Here's how the part is built. I have some questions about the finished solid (model axes, mm). Round coordinates to 2 decimals unless told otherwise and drop trailing zeros. Order: outer loops, then holes, each group sorted by start corner. A loop starts at its lowest first (then second) coordinate and runs counter-clockwise, first axis right, second up. Notation, with made-up numbers: M 85,-19 L 89,-19 A24 ccw 89,10 Z; hole C 84,53.25 d11. An arc over 180 degrees is marked long. Answer as CSV lines item,"result". Start each with the question number.
```python
from build123d import *

# Parameters (mm, degrees)
SKETCH1_W               = 283
SKETCH1_H               = 135
SKETCH1_R               = 1.75
BOSS_EXTRUDE1_DEPTH     = 4.5
SKETCH1_3_R             = 1.75
CUT_EXTRUDE1_DEPTH      = 4.5
MIRROR3_COPY_1_SKETCH_R = 1.75
MIRROR3_COPY_1_DEPTH    = 4.5
CUT_EXTRUDE2_REACH      = 6.5
SKETCH2_R               = 1.75
CUT_EXTRUDE3_REACH      = 6.5
SKETCH3_R               = 32.95
SKETCH3_R_2             = 14.5
SKETCH3_R_3             = 2.5


with BuildPart() as part:
    # Sketch1 → Boss-Extrude1 (new body)
    with BuildSketch(Plane.XY):
        Rectangle(SKETCH1_W, SKETCH1_H)
        with Locations((-131.5, 57.5)):
            Circle(SKETCH1_R, mode=Mode.SUBTRACT)
        with Locations((-131.5, 57.5)):
            Circle(SKETCH1_R)
    extrude(amount=BOSS_EXTRUDE1_DEPTH)

    # Sketch1_3 → Cut-Extrude1 (cut)
    with BuildSketch(Plane.XY):
        with Locations((-131.5, 57.5)):
            Circle(SKETCH1_3_R)
    cut_extrude1 = extrude(amount=CUT_EXTRUDE1_DEPTH, mode=Mode.SUBTRACT)

    # Mirror2: Cut-Extrude1 across plane
    add(cut_extrude1.mirror(Plane.ZX), mode=Mode.SUBTRACT)

    # Mirror3: Cut-Extrude1 across plane
    add(cut_extrude1.mirror(Plane(origin=(0, 0, 0), x_dir=(0, 0, 1), z_dir=(1, 0, 0))), mode=Mode.SUBTRACT)

    # Mirror3 copy 1 sketch → Mirror3 copy 1 (cut)
    with BuildSketch(Plane(origin=(0, 0, 0), x_dir=(-1, 0, 0), z_dir=(0, 0, 1))):
        with Locations((-131.5, 57.5)):
            Circle(MIRROR3_COPY_1_SKETCH_R)
    extrude(amount=MIRROR3_COPY_1_DEPTH, mode=Mode.SUBTRACT)

    # Sketch2 → Cut-Extrude2 (cut, up to next)
    with BuildSketch(Plane.XY.offset(4.5), mode=Mode.PRIVATE) as cut_extrude2_sk1:
        with Locations((-87.5, -14)):
            Circle(SKETCH2_R)
    cut_extrude2_tool1 = extrude(cut_extrude2_sk1.sketch, amount=-CUT_EXTRUDE2_REACH, mode=Mode.PRIVATE) & part.part
    add(cut_extrude2_tool1.solids().sort_by_distance((-87.5, -14, 4.5))[0], mode=Mode.SUBTRACT)
    # Sketch2 → Cut-Extrude2 (cut, up to next)
    with BuildSketch(Plane.XY.offset(4.5), mode=Mode.PRIVATE) as cut_extrude2_sk2:
        with Locations((-115.5, -14)):
            Circle(SKETCH2_R)
    cut_extrude2_tool2 = extrude(cut_extrude2_sk2.sketch, amount=-CUT_EXTRUDE2_REACH, mode=Mode.PRIVATE) & part.part
    add(cut_extrude2_tool2.solids().sort_by_distance((-115.5, -14, 4.5))[0], mode=Mode.SUBTRACT)
    # Sketch2 → Cut-Extrude2 (cut, up to next)
    with BuildSketch(Plane.XY.offset(4.5), mode=Mode.PRIVATE) as cut_extrude2_sk3:
        with Locations((-115.5, 14)):
            Circle(SKETCH2_R)
    cut_extrude2_tool3 = extrude(cut_extrude2_sk3.sketch, amount=-CUT_EXTRUDE2_REACH, mode=Mode.PRIVATE) & part.part
    add(cut_extrude2_tool3.solids().sort_by_distance((-115.5, 14, 4.5))[0], mode=Mode.SUBTRACT)
    # Sketch2 → Cut-Extrude2 (cut, up to next)
    with BuildSketch(Plane.XY.offset(4.5), mode=Mode.PRIVATE) as cut_extrude2_sk4:
        with Locations((-87.5, 14)):
            Circle(SKETCH2_R)
    cut_extrude2_tool4 = extrude(cut_extrude2_sk4.sketch, amount=-CUT_EXTRUDE2_REACH, mode=Mode.PRIVATE) & part.part
    add(cut_extrude2_tool4.solids().sort_by_distance((-87.5, 14, 4.5))[0], mode=Mode.SUBTRACT)
    # Sketch2 → Cut-Extrude2 (cut, up to next)
    with BuildSketch(Plane.XY.offset(4.5), mode=Mode.PRIVATE) as cut_extrude2_sk5:
        with BuildLine():
            Line((-68.5, -5), (-68.5, 5))
            ThreePointArc((-68.5, 5), (-66.5, 7), (-64.5, 5))
            Line((-64.5, 5), (-64.5, -5))
            ThreePointArc((-64.5, -5), (-66.5, -7), (-68.5, -5))
        make_face()
    cut_extrude2_tool5 = extrude(cut_extrude2_sk5.sketch, amount=-CUT_EXTRUDE2_REACH, mode=Mode.PRIVATE) & part.part
    add(cut_extrude2_tool5.solids().sort_by_distance((-66.5, 0, 4.5))[0], mode=Mode.SUBTRACT)

    # Sketch3 → Cut-Extrude3 (cut, up to next)
    with BuildSketch(Plane.XY.offset(4.5), mode=Mode.PRIVATE) as cut_extrude3_sk1:
        with Locations((75, -2.5)):
            Circle(SKETCH3_R)
    cut_extrude3_tool1 = extrude(cut_extrude3_sk1.sketch, amount=-CUT_EXTRUDE3_REACH, mode=Mode.PRIVATE) & part.part
    add(cut_extrude3_tool1.solids().sort_by_distance((75, -2.5, 4.5))[0], mode=Mode.SUBTRACT)
    # Sketch3 → Cut-Extrude3 (cut, up to next)
    with BuildSketch(Plane.XY.offset(4.5), mode=Mode.PRIVATE) as cut_extrude3_sk2:
        Circle(SKETCH3_R_2)
    cut_extrude3_tool2 = extrude(cut_extrude3_sk2.sketch, amount=-CUT_EXTRUDE3_REACH, mode=Mode.PRIVATE) & part.part
    add(cut_extrude3_tool2.solids().sort_by_distance((0, 0, 4.5))[0], mode=Mode.SUBTRACT)
    # Sketch3 → Cut-Extrude3 (cut, up to next)
    with BuildSketch(Plane.XY.offset(4.5), mode=Mode.PRIVATE) as cut_extrude3_sk3:
        with Locations((-6.525, -30.95)):
            Circle(SKETCH3_R_3)
    cut_extrude3_tool3 = extrude(cut_extrude3_sk3.sketch, amount=-CUT_EXTRUDE3_REACH, mode=Mode.PRIVATE) & part.part
    add(cut_extrude3_tool3.solids().sort_by_distance((-6.525, -30.95, 4.5))[0], mode=Mode.SUBTRACT)
    # Sketch3 → Cut-Extrude3 (cut, up to next)
    with BuildSketch(Plane.XY.offset(4.5), mode=Mode.PRIVATE) as cut_extrude3_sk4:
        with Locations((6.525, -30.95)):
            Circle(SKETCH3_R_3)
    cut_extrude3_tool4 = extrude(cut_extrude3_sk4.sketch, amount=-CUT_EXTRUDE3_REACH, mode=Mode.PRIVATE) & part.part
    add(cut_extrude3_tool4.solids().sort_by_distance((6.525, -30.95, 4.5))[0], mode=Mode.SUBTRACT)


solid = part.part
```
Item 1: If I drill on line 1 along Y through (x, z) = (-131.5, 1.75); line 2 along Y through (x, z) = (-115.5, 1.85); line 3 along X through (y, z) = (-57.5, 0.9), over which ranges is the centre line in solid material (lowest first)?
Item 2: If we section it at C-C on z = 2.8: Count the separate pieces of the cut face and the enclosed holes in it, and give its area (3 significant figures).
Item 3: We'd pull the mould along X, two halves only. Please class faces 1 (the cylindrical face through (-7.07, -33.39, 2.28)), 2 (the cylindrical face through (5.98, -33.39, 2.28)), 3 (the flat face through (-2, 16, 0)): pulls with the +X half, pulls with the -X half, needs draft (parallel to the pull), parting line crosses it, or undercut.
Item 4: If we section it at A-A on x = 0: Please give me the cut outline in (y, z), and give its area (3 significant figures).
Item 5: For P1, Ø3, axis at x = -131.5, y = 57.5, coming from the +Z side, with a flat end and sliding along its axis, tell me the tip position at first contact or that it passes through.
Item 6: If we section it at B-B on y = 23: Please give me the cut outline in (x, z), and give its area (3 significant figures).
Geometry says:
1,line 1,"-67.5 to -59.25, -55.75 to 55.75, 59.25 to 67.5"
1,line 2,"-67.5 to -15.75, -12.25 to 12.25, 15.75 to 67.5"
1,line 3,"-141.5 to -133.25, -129.75 to 129.75, 133.25 to 141.5"
2,separate pieces,"1"
2,enclosed holes,"13"
2,area,"34,000 mm²"
3,face 1,"undercut"
3,face 2,"undercut"
3,face 3,"needs draft"
4,outline,"M -67.5,0 L -14.5,0 L -14.5,4.5 L -67.5,4.5 Z; M 14.5,0 L 67.5,0 L 67.5,4.5 L 14.5,4.5 Z"
4,area,"477 mm²"
5,P1,"through"
6,outline,"M -141.5,0 L 54.13,0 L 54.13,4.5 L -141.5,4.5 Z; M 95.87,0 L 141.5,0 L 141.5,4.5 L 95.87,4.5 Z"
6,area,"1,090 mm²"
